Build history of the part. All positions in model axes, mm. Round coordinates to 2 decimals unless told otherwise and drop trailing zeros. Loops run counter-clockwise (first coordinate to the right, second up) from the corner with the lowest first, then second, coordinate; pieces in that order, holes last. Notation, with made-up numbers: (43, -31) - (75, -31) arc R11 ccw to (75, -14) - close; hole circle Ø6 at (88, 60). An arc over 180 degrees is marked (long way). Use one line per item in the form item = value. Start each with the question number.
Q1. Saw through at C-C (x = -32). Give the cut face in (y, z) (3 decimals), then the cut area to 3 significant figures.
Q2. Saw through at B-B (x = 0). Count the separate pieces of the cut face and the enclosed holes in it, then the cut area to 3 significant figures.
Q3. Pin check, flat tips, straight feed: pin 1 (12.5 mm diameter, centred on x = 0, y = 104.54, fed in from +Z); pin 2 (1.9 mm diameter, centred on x = -1.5, z = 4, fed in from -Y); pin 3 (1.9 mm diameter, centred on x = 93.5, z = 4.5, fed in from -Y); pin 4 (1.9 mm diameter, centred on y = 91, z = 4, fed in from -X). Stop position of each tip, or through.
Q4. Drill centre lines: line 1 (X direction, y = -29.5, z = 1.75); line 2 (X direction, y = -67.5, z = 0.5); line 3 (X direction, y = 48.5, z = 5). Where is each one in solid material? Low to high.
Q5. Saw through at A-A (y = 18). Give the cut face in (x, z), then the cut area to 3 significant figures.
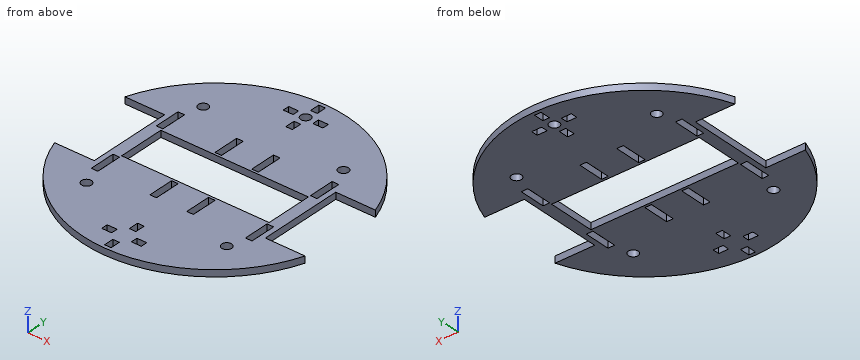
```python
from build123d import *

# Parameters (mm, degrees)
BOSS_EXTRUDE1_DEPTH     = 6.35
CUT_EXTRUDE1_DEPTH      = 176.071306912
CUT_EXTRUDE1_DEPTH_BACK = 176.071306912
SKETCH2_W               = 6.35
SKETCH2_H               = 24.999999975
SKETCH2_H_2             = 24.999999974
CUT_EXTRUDE2_DEPTH      = 176.071306912
CUT_EXTRUDE2_DEPTH_BACK = 176.071306912
SKETCH5_W               = 141.771062044
SKETCH5_H               = 45.249999988
CUT_EXTRUDE3_DEPTH      = 176.071306912
CUT_EXTRUDE3_DEPTH_BACK = 176.071306912
SKETCH6_R               = 4.7625
CUT_EXTRUDE4_DEPTH      = 176.071306912
CUT_EXTRUDE4_DEPTH_BACK = 176.071306912
SKETCH7_R               = 4.7625
CUT_EXTRUDE5_DEPTH      = 176.071306912
CUT_EXTRUDE5_DEPTH_BACK = 176.071306912
SKETCH8_W               = 6.35
SKETCH8_H               = 9.525
SKETCH8_W_2             = 9.525
SKETCH8_H_2             = 6.35


with BuildPart() as part:
    # Sketch1 → Boss-Extrude1 (new body)
    with BuildSketch(Plane.XY):
        with BuildLine():
            Line((120.335530928, -40.599999953), (82.235530928, -40.599999953))
            Line((82.235530928, -40.599999953), (82.235530928, 40.599999953))
            Line((82.235530928, 40.599999953), (120.335530928, 40.599999953))
            ThreePointArc((120.335530928, 40.599999953), (0, 127), (-120.335530928, 40.599999953))
            Line((-120.335530928, 40.599999953), (-82.235530928, 40.599999953))
            Line((-82.235530928, 40.599999953), (-82.235530928, -40.599999953))
            Line((-82.235530928, -40.599999953), (-120.335530928, -40.599999953))
            ThreePointArc((-120.335530928, -40.599999953), (0, -127), (120.335530928, -40.599999953))
        make_face()
    extrude(amount=BOSS_EXTRUDE1_DEPTH)

    # Sketch2 → Cut-Extrude1 (cut, two sides: drawn at the far end of the back side and taken through both)
    with BuildSketch(Plane.XY.offset(6.35).offset(-CUT_EXTRUDE1_DEPTH_BACK)):
        with Locations((17.710530946, 37.499999962)):
            Rectangle(SKETCH2_W, SKETCH2_H)
        with Locations((-74.060531022, 37.499999962)):
            Rectangle(SKETCH2_W, SKETCH2_H)
        with Locations((-17.710530946, 37.499999962)):
            Rectangle(SKETCH2_W, SKETCH2_H)
        with Locations((74.060531022, 37.499999962)):
            Rectangle(SKETCH2_W, SKETCH2_H_2)
        with Locations((74.060531022, -37.499999962)):
            Rectangle(SKETCH2_W, SKETCH2_H_2)
        with Locations((17.710530946, -37.499999962)):
            Rectangle(SKETCH2_W, SKETCH2_H)
        with Locations((-17.710530946, -37.499999962)):
            Rectangle(SKETCH2_W, SKETCH2_H_2)
        with Locations((-74.060531022, -37.499999962)):
            Rectangle(SKETCH2_W, SKETCH2_H_2)
    extrude(amount=CUT_EXTRUDE1_DEPTH + CUT_EXTRUDE1_DEPTH_BACK, mode=Mode.SUBTRACT)

    # Sketch5 → Cut-Extrude2 (cut, two sides: drawn at the far end of the back side and taken through both)
    with BuildSketch(Plane.XY.offset(6.35).offset(-CUT_EXTRUDE2_DEPTH_BACK)):
        Rectangle(SKETCH5_W, SKETCH5_H)
    extrude(amount=CUT_EXTRUDE2_DEPTH + CUT_EXTRUDE2_DEPTH_BACK, mode=Mode.SUBTRACT)

    # Sketch6 → Cut-Extrude3 (cut, two sides: drawn at the far end of the back side and taken through both)
    with BuildSketch(Plane.XY.offset(6.35).offset(-CUT_EXTRUDE3_DEPTH_BACK)):
        with Locations((-67.351920908, 67.351920908)):
            Circle(SKETCH6_R)
        with Locations((67.351920908, 67.351920908)):
            Circle(SKETCH6_R)
        with Locations((67.351920908, -67.351920908)):
            Circle(SKETCH6_R)
        with Locations((-67.351920908, -67.351920908)):
            Circle(SKETCH6_R)
    extrude(amount=CUT_EXTRUDE3_DEPTH + CUT_EXTRUDE3_DEPTH_BACK, mode=Mode.SUBTRACT)

    # Sketch7 → Cut-Extrude4 (cut, two sides: drawn at the far end of the back side and taken through both)
    with BuildSketch(Plane.XY.offset(6.35).offset(-CUT_EXTRUDE4_DEPTH_BACK)):
        with Locations((0, 104.537500094)):
            Circle(SKETCH7_R)
    extrude(amount=CUT_EXTRUDE4_DEPTH + CUT_EXTRUDE4_DEPTH_BACK, mode=Mode.SUBTRACT)

    # Sketch8 → Cut-Extrude5 (cut, two sides: drawn at the far end of the back side and taken through both)
    with BuildSketch(Plane.XY.offset(6.35).offset(-CUT_EXTRUDE5_DEPTH_BACK)):
        with Locations((0, 118.825000094)):
            Rectangle(SKETCH8_W, SKETCH8_H)
        with Locations((0, 90.250000094)):
            Rectangle(SKETCH8_W, SKETCH8_H)
        with Locations((0, -90.250000094)):
            Rectangle(SKETCH8_W, SKETCH8_H)
        with Locations((0, -118.825000094)):
            Rectangle(SKETCH8_W, SKETCH8_H)
        with Locations((-14.2875, 104.683652736)):
            Rectangle(SKETCH8_W_2, SKETCH8_H_2)
        with Locations((14.2875, 104.683652736)):
            Rectangle(SKETCH8_W_2, SKETCH8_H_2)
        with Locations((14.2875, -104.683652736)):
            Rectangle(SKETCH8_W_2, SKETCH8_H_2)
        with Locations((-14.2875, -104.683652736)):
            Rectangle(SKETCH8_W_2, SKETCH8_H_2)
    extrude(amount=CUT_EXTRUDE5_DEPTH + CUT_EXTRUDE5_DEPTH_BACK, mode=Mode.SUBTRACT)


solid = part.part
```
Report:
q1.outline = (-122.902, 0) - (-22.625, 0) - (-22.625, 6.35) - (-122.902, 6.35) - close; (22.625, 0) - (122.902, 0) - (122.902, 6.35) - (22.625, 6.35) - close
q1.area = 1,270 mm²
q2.separate_pieces = 7
q2.enclosed_holes = 0
q2.area = 1,020 mm²
q3.pin_1 = 6.35
q3.pin_2 = -127
q3.pin_3 = -86.97
q3.pin_4 = -89.55
q4.line_1 = -82.24 to -77.24, -70.89 to -20.89, -14.54 to 14.54, 20.89 to 70.89, 77.24 to 82.24
q4.line_2 = -107.58 to -72.11, -62.59 to 62.59, 72.11 to 107.58
q4.line_3 = -117.37 to -77.24, -70.89 to -20.89, -14.54 to 14.54, 20.89 to 70.89, 77.24 to 117.37
q5.outline = (-82.24, 0) - (-70.89, 0) - (-70.89, 6.35) - (-82.24, 6.35) - close; (70.89, 0) - (82.24, 0) - (82.24, 6.35) - (70.89, 6.35) - close
q5.area = 144 mm²
